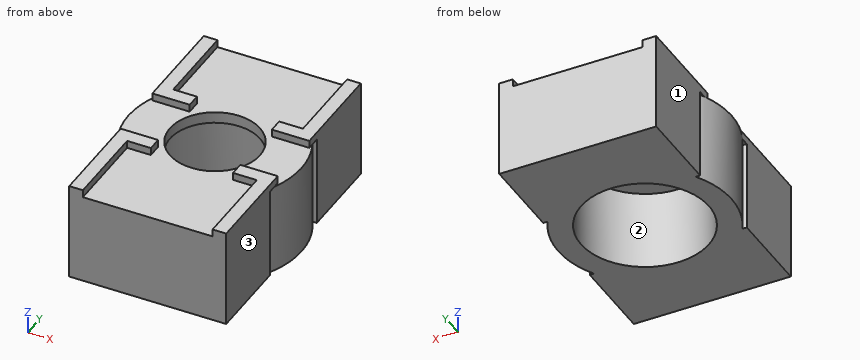
Autodesk Inventor part; units mm, degrees
ref_plane "YZ Plane" through (0, 0, 0) normal (1, 0, 0) x (0, 1, 0)
ref_plane "XZ Plane" through (0, 0, 0) normal (0, 1, 0) x (-1, 0, 0)
ref_plane "XY Plane" through (0, 0, 0) normal (0, 0, 1) x (1, 0, 0)
sketch "Sketch1" plane through (0, 0, 0) normal (0, 0, 1) x (1, 0, 0)
  circle A0 centre (0, 0) radius 7.925
  circle A1 centre (0, 0) radius 8.425
  point P0 (0, 0)
  dimension "d0" = 0.5
extrude "Extrusion1" add sketch "Sketch1" along normal blind 1.5 contours A0 | A1
sketch "Sketch2" plane through (0, 0, 1.5) normal (0, 0, 1) x (1, 0, 0)
  circle A0 centre (0, 0) radius 8.425
  circle A1 centre (0, 0) radius 11.425
  dimension "d3" = 3
extrude "Extrusion2" add sketch "Sketch2" against normal blind 12
sketch "Sketch3" plane through (0, 0, 1.5) normal (0, 0, 1) x (1, 0, 0)
  circle A0 centre (0, 0) radius 6.94
  circle A1 centre (0, 0) radius 5.94
  dimension "d6" = 1
extrude "Extrusion3" cut sketch "Sketch3" against normal through all contours A1
sketch "Sketch4" plane through (0, 0, 1.5) normal (0, 0, 1) x (1, 0, 0)
  line L0 (-8.355, 16.96) -> (-8.355, 7.9)
  line L1 (8.355, 7.9) -> (8.355, 16.96)
  line L2 (-10.355, 17.0459) -> (10.355, 17.0459)
  line L3 (10.355, 17.0459) -> (10.355, 5.9)
  line L4 (-10.355, 5.9) -> (-10.355, 17.0459)
  circle A0 centre (0, 0) radius 10.575
  line L5 (-8.7761, 5.9) -> (-10.355, 5.9)
  line L6 (10.355, 5.9) -> (8.7761, 5.9)
  arc A1 (8.7761, 5.9) -> (-8.7761, 5.9) centre (0, 0) ccw
extrude "Extrusion4" add sketch "Sketch4" against normal up to surface (12 mm away) contours L2 L3 L6 A0 L5 L4
sketch "Sketch5" plane through (0, 0, 1.5) normal (0, 0, 1) x (1, 0, 0)
  line L0 (10.355, 17.0459) -> (-10.355, 17.0459)
  line L1 (-8.355, 16.96) -> (-8.355, 7.9)
  line L2 (8.355, 7.9) -> (8.355, 16.96)
  line L3 (-6.395, 5.94) -> (6.395, 5.94)
  line L4 (-8.555, 17.0459) -> (-8.555, 7.9)
  line L5 (-8.555, 7.9) -> (-8.555, 5.94)
  line L6 (-8.555, 5.94) -> (-8.555, 5.84)
  line L7 (-8.555, 5.84) -> (-5.4211, 5.84)
  line L8 (-5.4211, 5.84) -> (-5.4211, 4.0009)
  line L9 (-5.4211, 4.0009) -> (-10.355, 4.0009)
  line L10 (-10.355, 4.0009) -> (-10.355, 17.0459)
  line L11 (-10.355, 17.0459) -> (-8.555, 17.0459)
  dimension "d12" = 0.2
  dimension "d13" = 0.1
extrude "Extrusion5" add sketch "Sketch5" along normal blind 1
sketch "Sketch6" plane through (0, 0, 2.5) normal (0, 0, 1) x (1, 0, 0)
  line L0 (-10.355, 4.0009) -> (-5.4211, 4.0009)
  line L1 (-5.4211, 4.0009) -> (-5.4211, 13.0009)
  line L2 (-5.4211, 13.0009) -> (-10.355, 13.0009)
  line L3 (-10.355, 13.0009) -> (-10.355, 4.0009)
  point P0 (0, 0)
  dimension "d18" = 9
extrude "Extrusion6" [suppressed]
mirror "Mirror1" about plane through (0, 0, 0) normal (1, 0, 0) of "Extrusion5"
mirror "Mirror2" about plane through (0, 0, 0) normal (0, 1, 0) of "Extrusion5", "Mirror1", "Extrusion4"
properties part number "PI_holder"
Build history of the part. All positions in model axes, mm. Face numbers are marked on the shaded views. Round coordinates to 2 decimals unless told otherwise and drop trailing zeros. Loops run counter-clockwise (first coordinate to the right, second up) from the corner with the lowest first, then second, coordinate; pieces in that order, holes last.
Item 1: Saw through at A-A (x = 0). List the corners of the cut face in (y, z) (3 decimals), then the cut area to 3 significant figures.
Item 2: Pin check, flat tips, straight feed: P1, Ø1, axis at y = -11.5, z = -2, coming from the -X side (3 decimals); P2, Ø5, axis at x = -1, y = 1.5, coming from the +Z side; P3, Ø0.8, axis at x = -7.5, z = 2, coming from the +Y side; P4, Ø1.1, axis at y = -13.5, z = 2, coming from the +X side (3 decimals). Stop position of each tip, or through.
Item 3: Saw through at C-C (z = -6.5). List the corners of the cut face in (x, y) (3 decimals).
Item 4: Two-plate mould, pull along X, no slides. Class the marked faces 1, 2 and 3: released by +X, released by -X, zero draft, split by the parting line, or undercut.
Item 5: Drill centre lines: line 1 along Y through (x, z) = (0, -7.5) (3 decimals); line 2 along Z through (x, y) = (8, -3.5); line 3 along X through (y, z) = (-9, 0.75) (3 decimals). Where is each one in solid material? Low to high.
Item 6: Saw through at B-B (y = 0). List the corners of the cut face in (x, z) (3 decimals).
Item 7: Saw through at D-D (y = -15). List the corners of the cut face in (x, z) (3 decimals).
Worked answers:
1. outline: (-17.046, -10.5) - (-8.425, -10.5) - (-8.425, 0) - (-5.94, 0) - (-5.94, 1.5) - (-17.046, 1.5) - close; (5.94, 0) - (8.425, 0) - (8.425, -10.5) - (17.046, -10.5) - (17.046, 1.5) - (5.94, 1.5) - close
1. area: 214 mm2
2. P1: stops at x = -10.355
2. P2: passes through
2. P3: stops at y = 5.84
2. P4: stops at x = 10.355
3. outline: (-10.355, -17.046) - (10.355, -17.046) - (10.355, -5.9) - (9.784, -5.9) arc R11.425 ccw to (9.784, 5.9) - (10.355, 5.9) - (10.355, 17.046) - (-10.355, 17.046) - (-10.355, 5.9) - (-9.784, 5.9) arc R11.425 ccw to (-9.784, -5.9) - (-10.355, -5.9) - close; hole circle Ø16.85 at (0, 0)
4. face 1: released by -X
4. face 2: undercut
4. face 3: released by +X
5. line 1: y = -17.046 to -8.425, 8.425 to 17.046
5. line 2: z = -10.5 to 1.5
5. line 3: x = -10.355 to 10.355
6. outline: (-11.425, -10.5) - (-8.425, -10.5) - (-8.425, 0) - (-5.94, 0) - (-5.94, 1.5) - (-11.425, 1.5) - close; (5.94, 0) - (8.425, 0) - (8.425, -10.5) - (11.425, -10.5) - (11.425, 1.5) - (5.94, 1.5) - close
7. outline: (-10.355, -10.5) - (10.355, -10.5) - (10.355, 2.5) - (8.555, 2.5) - (8.555, 1.5) - (-8.555, 1.5) - (-8.555, 2.5) - (-10.355, 2.5) - close
